Input: part model. Units: mm. Frame: model coordinates. Face numbers are marked on the shaded views. A direction names the side the tool comes from. Give positions to 0.01 mm unless a question says otherwise; leave off trailing zeros. Loops run counter-clockwise (first coordinate to the right, second up) from the corner with the lowest first, then second, coordinate; pieces in that order, holes last. Notation, with made-up numbers: (-1.75, 64) - (13.25, 64) arc R20 ccw to (13.25, 80) - close; hole circle Ø7 at (67, 79.25). An arc over 180 degrees is marked (long way). One line per item, written item: value.
from build123d import *

# Parameters (mm, degrees)
CROQUIS1_W                 = 5
CROQUIS1_H                 = 13
SALIENTE_EXTRUIR1_DEPTH    = 3
CROQUIS9_R                 = 3.9
SALIENTE_EXTRUIR2_DEPTH    = 30
CROQUIS10_R                = 2
CORTAR_EXTRUIR7_DEPTH      = 27.5
CORTAR_EXTRUIR7_DEPTH_BACK = 27.5


with BuildPart() as part:
    # Croquis1 → Saliente-Extruir1 (new body)
    with BuildSketch(Plane(origin=(0, 0, 0), x_dir=(1, 0, 0), z_dir=(0, 1, 0))):
        Polygon((-45, -26.5), (-30, -26.5), (0, -18.5), (30, -26.5), (45, -26.5), (45, -7.5), (30, -7.5), (22, 0), (30, 7.5), (45, 7.5), (45, 26.5), (30, 26.5), (0, 18.5), (-30, 26.5), (-45, 26.5), (-45, 7.5), (-30, 7.5), (-22, 0), (-30, -7.5), (-45, -7.5), align=None)
        with Locations((39.5, -17)):
            Rectangle(CROQUIS1_W, CROQUIS1_H, mode=Mode.SUBTRACT)
        with Locations((39.5, 17)):
            Rectangle(CROQUIS1_W, CROQUIS1_H, mode=Mode.SUBTRACT)
        with Locations((-39.5, 17)):
            Rectangle(CROQUIS1_W, CROQUIS1_H, mode=Mode.SUBTRACT)
        with Locations((-39.5, -17)):
            Rectangle(CROQUIS1_W, CROQUIS1_H, mode=Mode.SUBTRACT)
    extrude(amount=SALIENTE_EXTRUIR1_DEPTH)

    # Croquis9 → Saliente-Extruir2 (add)
    with BuildSketch(Plane(origin=(0, 3, 0), x_dir=(1, 0, 0), z_dir=(0, 1, 0))):
        Circle(CROQUIS9_R)
    extrude(amount=SALIENTE_EXTRUIR2_DEPTH)

    # Croquis10 → Cortar-Extruir7 (cut, two sides)
    with BuildSketch(Plane.XY) as cortar_extruir7_sk:
        with Locations((0, 30)):
            Circle(CROQUIS10_R)
    extrude(amount=CORTAR_EXTRUIR7_DEPTH, mode=Mode.SUBTRACT)
    extrude(cortar_extruir7_sk.sketch, amount=-CORTAR_EXTRUIR7_DEPTH_BACK, mode=Mode.SUBTRACT)


solid = part.part
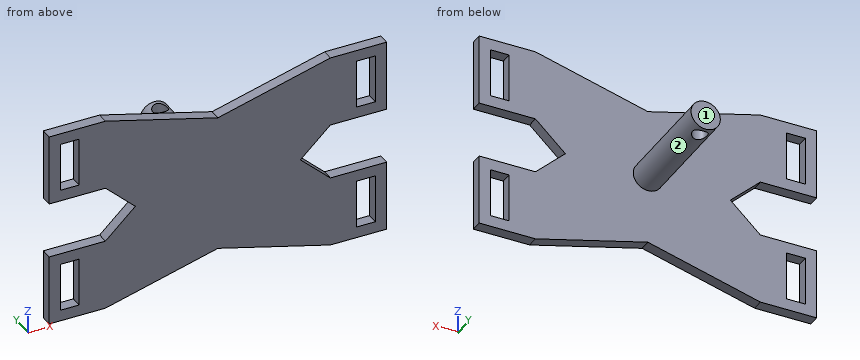
Item 1: Section D-D, the plane x = 12. Output: boundary loops of the cut face in (y, z).
Verdict:
outline: (0, -21.7) - (3, -21.7) - (3, 21.7) - (0, 21.7) - close
Item 2: Material intervals for L1, parallel to Y at x = 0, z = 0; L2, parallel to X at y = 30, z = 0.25; L3, parallel to Y at x = -39, z = -8.5, sorted ascending.
Verdict:
L1: y = 0 to 28, 32 to 33
L2: x = -3.89 to -2, 2 to 3.89
L3: y = 0 to 3
Item 3: Section C-C, the plane y = 30. Output: boundary loops of the cut face in (x, z), and give its area (3 significant figures).
Verdict:
outline: (-2, -3.35) - (-2, 3.35) arc R3.9 ccw to start; (2, -3.35) arc R3.9 ccw to (2, 3.35) - close
area: 18.0 mm^2
Item 4: Pin query (flat end, axial travel): P1, Ø3, axis at x = -17, z = -12, coming from the +Y side; P2, Ø2.5, axis at x = 0, y = 30, coming from the -Z side; P3, Ø1, axis at x = 2.5, y = 7, coming from the +Z side; P4, Ø10, axis at x = -1, y = 19.5, coming from the +Z side. Return the tip coordinate at first contact, or that it passes through.
Verdict:
P1: stops at y = 3
P2: passes through
P3: stops at z = 3.35
P4: stops at z = 3.9
Item 5: Access query for the marked faces 1 and 2. Directions: +Z, -Z, +X, -X, +Y, -Y. A direction counts if a zero-diameter tool reaches every point of the face in a straight line with its end or side. Return the directions, or none.
Verdict:
face 1: +Z, -Z, +X, -X, +Y
face 2: +Y
Item 6: Section B-B, the plane y = 22. Output: boundary loops of the cut face in (x, z).
Verdict:
outline: circle Ø7.8 at (0, 0)
Item 7: Section A-A, the plane z = 12. Output: boundary loops of the cut face in (x, y).
Verdict:
outline: (-45, 0) - (-42, 0) - (-42, 3) - (-45, 3) - close; (-37, 0) - (37, 0) - (37, 3) - (-37, 3) - close; (42, 0) - (45, 0) - (45, 3) - (42, 3) - close
